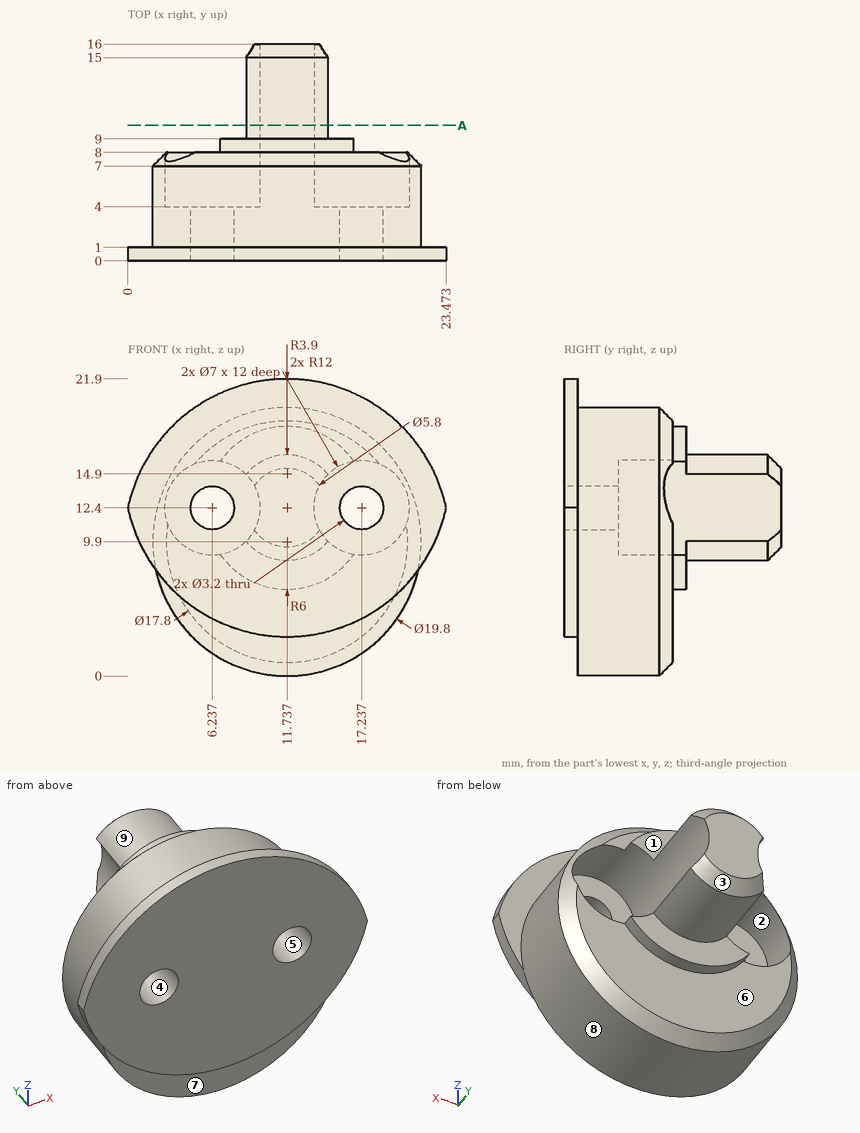
Study the drawing (mm; zero at the part's minimum x, y, z) and answer. A direction names the side the tool comes from. Give positions to 0.01 mm unless a question says otherwise; leave off trailing zeros. Loops run counter-clockwise (first coordinate to the right, second up) from the corner with the lowest first, then second, coordinate; pieces in that order, holes last. Notation, with made-up numbers: (-32.5, 45) -> (-9.5, 45) arc R26 ccw to (-9.5, 74) -> close; hole circle Ø6 at (8, 50.25). An arc over 180 degrees is marked (long way). Write item = value, one per line. Start each with the question number.
(1) Which of the six approach directions +Z, -Z, +X, -X, +Y, -Y give full straight-line access (tool end or side, diameter ignored) to the marked faces 5, 6, 7, 8 and 9?
(2) Given pin 1 Ø11.5 at (x, z) = (11.5, 7.5) entering from +Y; pin 2 Ø3.5 at (x, z) = (6.5, 11) entering from +Y; pin 3 Ø3 at (x, y) = (5, 3.5) entering from -Z; pin 4 Ø4 at (x, z) = (11, 17.5) entering from +Y, each flat-ended and moving along its own axis, determine where each tip first touches the part or whether it passes through.
(3) The mould has two halves that part along Z. Classify the marked faces 1, 2, 3 and 4: +Z half, -Z half, draft (parallel to the pull), parting line (faces both ways), or undercut.
(4) Find the intervals of material crossed by probe 1 along X at (y, z) = (1.65, 12.4) (1 decimal); probe 2 along Y at (x, z) = (4, 9); probe 3 along Y at (x, z) = (16.75, 20.5), in increasing order. Write a range as from..to.
(5) Find section A-A on y = 10. Give the vertices of the cut face in (x, z) (1 decimal).
From the geometry:
q1.face_5 = +Y, -Y
q1.face_6 = -Z, +Y
q1.face_7 = -Z, -Y
q1.face_8 = +Y
q1.face_9 = +Z, +Y
q2.pin_1 = 16
q2.pin_2 = 4
q2.pin_3 = 1.5
q2.pin_4 = 15.75
q3.face_1 = draft
q3.face_2 = undercut
q3.face_3 = -Z half
q3.face_4 = undercut
q4.probe_1 = 2.2..4.6, 7.8..15.6, 18.8..21.3
q4.probe_2 = 0..8
q4.probe_3 = 0..1
q5.outline = (8.7, 9.9) arc R3.9 ccw to (14.8, 9.9) arc R3.5 cw to (14.8, 14.9) arc R3.9 ccw to (8.7, 14.9) arc R3.5 cw to start
